Source: CAD feature listing. Evaluate the final solid. Frame: model axes, mm. Give positions to 0.01 mm unless a question says otherwise; leave off trailing zeros. Order: outer loops, then holes, each group sorted by start corner. A loop starts at its lowest first (then second) coordinate and runs counter-clockwise, first axis right, second up. Notation, with made-up numbers: (19, -26.75) - (52, -26.75) arc R25 ccw to (52, -8.75) - close; hole circle Ø2 at (9.5, -11.75). An arc over 180 degrees is marked (long way). Answer as CSV lines item,"result".
```python
from build123d import *

# Parameters (mm, degrees)
SKETCH1_R           = 3.175
BOSS_EXTRUDE1_DEPTH = 3.175
FILLET2_R           = 6.35


with BuildPart() as part:
    # Sketch1 → Boss-Extrude1 (new body)
    with BuildSketch(Plane(origin=(0, 0, 0), x_dir=(0, 0, -1), z_dir=(1, 0, 0))):
        Polygon((31.75, 0), (16.51, 30.48), (6.35, 30.48), (0, 0), align=None)
        with Locations((11.43, 23.92807)):
            Circle(SKETCH1_R, mode=Mode.SUBTRACT)
    extrude(amount=BOSS_EXTRUDE1_DEPTH)

    # Fillet2
    fillet2_edges = [part.edges().sort_by_distance(p)[0] for p in [
        (1.5875, 30.48, -6.35),
        (1.5875, 30.48, -16.51),
    ]]
    fillet(fillet2_edges, radius=FILLET2_R)


solid = part.part
```
(1) Ray query, line 1 (Y direction, x = 1.8, z = -11.43); line 2 (Z direction, x = 2.15, y = 25); line 3 (Y direction, x = 1.9, z = -9.5). Return the intervals inside material, ascending. Write a range as from..to.
Completed:
line 1,"0..20.75, 27.1..30.48"
line 2,"-19.25..-14.42, -8.44..-5.21"
line 3,"0..21.41, 26.45..30.15"
(2) Cut plane A-A (z = -13). Return loops of the section in (x, y) (3 decimals), then the cut area to 3 significant figures.
Completed:
outline,"(0, 0) - (3.175, 0) - (3.175, 21.168) - (0, 21.168) - close; (0, 26.688) - (3.175, 26.688) - (3.175, 30.466) - (0, 30.466) - close"
area,"79.2 mm²"
(3) Cut plane D-D (z = -23). Return loops of the section in (x, y) (3 decimals).
Completed:
outline,"(0, 0) - (3.175, 0) - (3.175, 17.5) - (0, 17.5) - close"
(4) Cut plane C-C (x = 1.9). Return loops of the section in (y, z) (3 decimals).
Completed:
outline,"(0, -31.75) - (26.97, -18.265) arc R6.35 ccw to (30.48, -12.585) - (30.48, -11.513) arc R6.35 ccw to (25.425, -5.297) - (0, 0) - close; hole circle Ø6.35 at (23.928, -11.43)"
(5) Mould query, pull axis Z, two halves, no side actions, for faces 1 (the flat face through (2, 30.48, -12)), 2 (the cylindrical face through (1.565, 27.076, -11.017)), 3 (the flat face through (1.565, 12.891, -2.686)), 4 (the cylindrical face through (1.61, 29.506, -15.966)). Classes: released by +Z, released by -Z, zero draft, split by the parting line, or undercut.
Completed:
face 1,"zero draft"
face 2,"undercut"
face 3,"released by +Z"
face 4,"released by -Z"
(6) Cut plane B-B (y = 26). Return loops of the section in (x, z) (3 decimals).
Completed:
outline,"(0, -18.75) - (3.175, -18.75) - (3.175, -13.836) - (0, -13.836) - close; (0, -9.024) - (3.175, -9.024) - (3.175, -5.445) - (0, -5.445) - close"
(7) Contact query for flat-ended pins moving along their axis: pin 1 (8 mm diameter, centred on y = 12.5, z = -28.5, fed in from +X) (3 decimals); pin 2 (1.5 mm diameter, centred on x = 1.5, y = 17.5, fed in from +Z); pin 3 (1.5 mm diameter, centred on x = 1.5, y = 20, fed in from +Z). Output: stop coordinate, or through.
Completed:
pin 1,"x = 3.175"
pin 2,"z = -3.49"
pin 3,"z = -4.01"
